Model file for the job. Use its own axes, mm. Face numbers are marked on the shaded views. A direction names the side the tool comes from. Give positions to 0.01 mm unless a question says otherwise; leave off trailing zeros. Loops run counter-clockwise (first coordinate to the right, second up) from the corner with the lowest first, then second, coordinate; pieces in that order, holes last. Notation, with made-up numbers: (10, -10.75) - (55, -10.75) arc R22 ccw to (55, 21.25) - close; hole circle Ø1 at (36, -4.75). An arc over 180 degrees is marked (long way). Use a Markdown table: item, result.
from build123d import *

# Parameters (mm, degrees)
SKETCH1_W           = 36.5
SKETCH1_H           = 18
BOSS_EXTRUDE1_DEPTH = 1.2
SKETCH2_W           = 3.6
SKETCH2_H           = 5
SKETCH2_W_2         = 4.8
SKETCH2_H_2         = 6
BOSS_EXTRUDE2_DEPTH = 4
CUT_EXTRUDE1_REACH  = 7.2
SKETCH3_W           = 10.5
SKETCH3_H           = 13.2
FILLET1_R           = 1


with BuildPart() as part:
    # Sketch1 → Boss-Extrude1 (new body)
    with BuildSketch(Plane(origin=(0, 0, 0), x_dir=(1, 0, 0), z_dir=(0, 1, 0))):
        with Locations((18.25, 9)):
            Rectangle(SKETCH1_W, SKETCH1_H)
    extrude(amount=BOSS_EXTRUDE1_DEPTH)

    # Sketch2 → Boss-Extrude2 (add)
    with BuildSketch(Plane.XZ):
        with Locations((3.8, -4.5)):
            Rectangle(SKETCH2_W, SKETCH2_H)
        with Locations((32.1, -5)):
            Rectangle(SKETCH2_W_2, SKETCH2_H_2)
    extrude(amount=BOSS_EXTRUDE2_DEPTH)

    # Sketch3 → Cut-Extrude1 (cut, up to next)
    with BuildSketch(Plane(origin=(0, 1.2, 0), x_dir=(1, 0, 0), z_dir=(0, 1, 0)), mode=Mode.PRIVATE) as cut_extrude1_sk1:
        with Locations((23.75, 9)):
            Rectangle(SKETCH3_W, SKETCH3_H)
    cut_extrude1_tool1 = extrude(cut_extrude1_sk1.sketch, amount=-CUT_EXTRUDE1_REACH, mode=Mode.PRIVATE) & part.part
    add(cut_extrude1_tool1.solids().sort_by_distance((23.75, 1.2, -9))[0], mode=Mode.SUBTRACT)

    # Fillet1
    fillet1_edges = [part.edges().sort_by_distance(p)[0] for p in [
        (18.5, 0.6, -2.4),
        (18.5, 0.6, -15.6),
        (29, 0.6, -15.6),
        (29, 0.6, -2.4),
    ]]
    fillet(fillet1_edges, radius=FILLET1_R)


solid = part.part
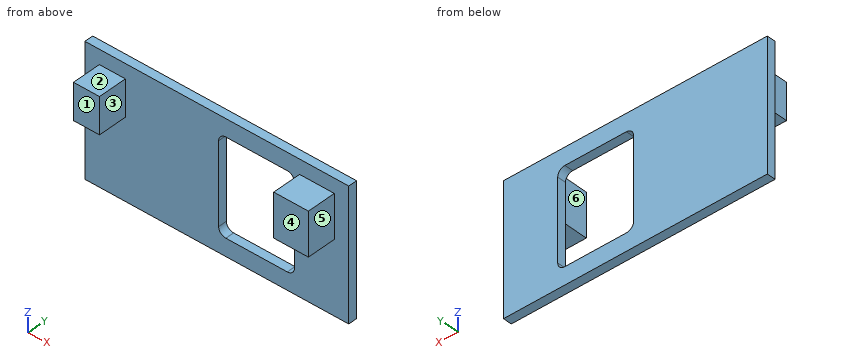
(1) Mould opens along X. For the marked faces 3, 4, 5 and 6 say: pulls with the +X half, pulls with the -X half, needs draft (parallel to the pull), parting line crosses it, or undercut.
Computed:
| item | result |
|---|---|
| face 3 | undercut |
| face 4 | needs draft |
| face 5 | pulls with the +X half |
| face 6 | undercut |
(2) Slice it at D-D, the plane z = -16.5. Write the cut outline in (x, y).
Computed:
| item | result |
|---|---|
| outline | (0, 0) - (36.5, 0) - (36.5, 1.2) - (0, 1.2) - close |
(3) 3-axis set-ups, long thin cutter, end or side, ignore diameter. For the marked faces 1 and 2: which of +Z, -Z, +X, -X, +Y, -Y reach the whole face in a straight line?
Computed:
| item | result |
|---|---|
| face 1 | +Z, -Z, +X, -X, -Y |
| face 2 | +Z, +X, -X, -Y |
(4) Slice it at A-A, the plane z = -10. Write the cut outline in (x, y).
Computed:
| item | result |
|---|---|
| outline | (0, 0) - (18.5, 0) - (18.5, 1.2) - (0, 1.2) - close; (29, 0) - (36.5, 0) - (36.5, 1.2) - (29, 1.2) - close |
(5) Slice it at B-B, the plane y = -2.2. Write the cut outline in (x, z).
Computed:
| item | result |
|---|---|
| outline | (2, -7) - (5.6, -7) - (5.6, -2) - (2, -2) - close; (29.7, -8) - (34.5, -8) - (34.5, -2) - (29.7, -2) - close |
(6) Pin check, flat tips, straight feed: P1, Ø2, axis at x = 17, y = -2, coming from the +Z side; P2, Ø1.1, axis at x = 3.5, y = -2.5, coming from the -Z side; P3, Ø1.2, axis at x = 32.5, y = -2, coming from the -Z side; P4, Ø1.2, axis at y = -1, z = -5.5, coming from the -X side. Stop position of each tip, or through.
Computed:
| item | result |
|---|---|
| P1 | through |
| P2 | z = -7 |
| P3 | z = -8 |
| P4 | x = 2 |
(7) Drill centre lines: probe 1 along X at (y, z) = (0.5, -13); probe 2 along X at (y, z) = (-2.65, -5); probe 3 along Y at (x, z) = (33.5, -1.5). Where is each one in solid material? Low to high. Write a range as [from, to].
Computed:
| item | result |
|---|---|
| probe 1 | [0, 18.5], [29, 36.5] |
| probe 2 | [2, 5.6], [29.7, 34.5] |
| probe 3 | [0, 1.2] |
(8) Slice it at C-C, the plane x = 4. Write the cut outline in (y, z), plus the area to 3 significant figures.
Computed:
| item | result |
|---|---|
| outline | (-4, -7) - (0, -7) - (0, -18) - (1.2, -18) - (1.2, 0) - (0, 0) - (0, -2) - (-4, -2) - close |
| area | 41.6 mm² |
